from build123d import *

# Parameters (mm, degrees)
SKETCH1_R           = 3.175
BOSS_EXTRUDE1_DEPTH = 3.175
SKETCH2_W           = 17.78
SKETCH2_H           = 4.7625
BOSS_EXTRUDE2_DEPTH = 10.16
SKETCH3_R           = 6.35
CUT_EXTRUDE1_DEPTH  = 17.78
FILLET2_R           = 1.27
FILLET3_R           = 1.27


with BuildPart() as part:
    # Sketch1 → Boss-Extrude1 (new body)
    with BuildSketch(Plane.XY):
        with BuildLine():
            Line((-8.89, 0), (-8.89, -10.16))
            Line((-8.89, -10.16), (8.89, -10.16))
            Line((8.89, -10.16), (8.89, 0))
            ThreePointArc((8.89, 0), (0, 8.89), (-8.89, 0))
        make_face()
        Circle(SKETCH1_R, mode=Mode.SUBTRACT)
    extrude(amount=BOSS_EXTRUDE1_DEPTH)

    # Sketch2 → Boss-Extrude2 (add)
    with BuildSketch(Plane.XY.offset(3.175)):
        with Locations((0, -7.77875)):
            Rectangle(SKETCH2_W, SKETCH2_H)
    extrude(amount=BOSS_EXTRUDE2_DEPTH)

    # Sketch3 → Cut-Extrude1 (cut)
    with BuildSketch(Plane(origin=(0, -10.16, 0), x_dir=(-1, 0, 0), z_dir=(0, -1, 0))):
        with Locations((0, -13.335)):
            Circle(SKETCH3_R)
    extrude(amount=-CUT_EXTRUDE1_DEPTH, mode=Mode.SUBTRACT)

    # Fillet2
    fillet2_edges = [part.edges().sort_by_distance(p)[0] for p in [
        (-8.89, -7.77875, 13.335),
        (8.89, -7.77875, 13.335),
    ]]
    fillet(fillet2_edges, radius=FILLET2_R)

    # Fillet3
    fillet3_edges = [part.edges().sort_by_distance(p)[0] for p in [
        (-6.35, -7.77875, 13.335),
        (6.35, -7.77875, 13.335),
    ]]
    fillet(fillet3_edges, radius=FILLET3_R)


solid = part.part
Geometry: final body of the model. Coordinates: model frame, mm. A direction names the side the tool comes from. Give positions to 0.01 mm unless a question says otherwise; leave off trailing zeros. Write each loop counter-clockwise with the first axis right and the second up, starting at its lowest first coordinate (ties: lowest second). Pieces come first, ordered by that corner, then holes. Notation, with made-up numbers: M -30,-27 L -5,-27 A26 ccw -5,8 Z; hole C 60,8 d7. An arc over 180 degrees is marked long. Answer in a Markdown table with one row per item. Add a question column.
(1) First-contact query: pin 1 (4 mm diameter, centred on x = -2.5, z = 2, fed in from +Y); pin 2 (5 mm diameter, centred on x = 0, y = 0.5, fed in from -Z); pin 3 (2 mm diameter, centred on x = 6.5, y = 2, fed in from +Z) (3 decimals). Flat tips, straight axial feed; report the tip coordinate or a pass-through.
(2) Section B-B on y = -1. Return loops of the section in (x, z) (3 decimals), and give its area (3 significant figures).
(3) Ray query, line 1 (Y direction, x = 3, z = 4.25); line 2 (Y direction, x = 0, z = 0.85) (3 decimals); line 3 (Z direction, x = -8, y = 2.5) (3 decimals). Return the intervals inside material, ascending.
(4) Mould query, pull axis Y, two halves, no side actions, for faces 4 (the cylindrical face through (-6.684, -7.745, 13.027)), 5 (the cylindrical face through (-0.69, -3.1, 1.57)), 6 (the flat face through (0, -10.16, 5)). Classes: +Y half, -Y half, draft (parallel to the pull), parting line (faces both ways), or undercut.
(5) Reachability of faces 1 (the flat face through (8.89, -7, 5)), 2 (the cylindrical face through (6.7, -7.81, 13.04)), 3 (the flat face through (-0.1, 3.4, 3.175)) from +Z, -Z, +X, -X, +Y, -Y: full face, straight path, thin tool, end or side. Return the list, or none.
(6) Section A-A on x = 0. Return loops of the section in (y, z) (1 decimal).
(7) Section C-C on z = 9.75. Return loops of the section in (x, y), and give its area (3 significant figures).
(8) Section D-D on x = 2.5. Return loops of the section in (y, z) (1 decimal), and give its area (3 significant figures).
Result set:
| question | item | result |
|---|---|---|
| 1 | pin 1 | stops at y = 8.88 |
| 1 | pin 2 | passes through |
| 1 | pin 3 | stops at z = 3.175 |
| 2 | outline | M -8.89,0 L -3.013,0 L -3.013,3.175 L -8.89,3.175 Z; M 3.013,0 L 8.89,0 L 8.89,3.175 L 3.013,3.175 Z |
| 2 | area | 37.3 mm^2 |
| 3 | line 1 | y = -10.16 to -5.4 |
| 3 | line 2 | y = -10.16 to -3.175, 3.175 to 8.89 |
| 3 | line 3 | z = 0 to 3.175 |
| 4 | face 4 | draft |
| 4 | face 5 | undercut |
| 4 | face 6 | -Y half |
| 5 | face 1 | +Z, -Z, +X, +Y, -Y |
| 5 | face 2 | +Z, +Y, -Y |
| 5 | face 3 | +Z, +X, -X, +Y |
| 6 | outline | M -10.2,0 L -3.2,0 L -3.2,3.2 L -5.4,3.2 L -5.4,7 L -10.2,7 Z; M 3.2,0 L 8.9,0 L 8.9,3.2 L 3.2,3.2 Z |
| 7 | outline | M -8.89,-10.16 L -5.24,-10.16 L -5.24,-5.4 L -8.89,-5.4 Z; M 5.24,-10.16 L 8.89,-10.16 L 8.89,-5.4 L 5.24,-5.4 Z |
| 7 | area | 34.8 mm^2 |
| 8 | outline | M -10.2,0 L -2,0 L -2,3.2 L -5.4,3.2 L -5.4,7.5 L -10.2,7.5 Z; M 2,0 L 8.5,0 L 8.5,3.2 L 2,3.2 Z |
| 8 | area | 67.5 mm^2 |
